Read the model definition and answer for the solid it produces. Units are mm, in the model's axes. Round coordinates to 2 decimals unless told otherwise and drop trailing zeros. Order: outer loops, then holes, each group sorted by start corner. A loop starts at its lowest first (then second) coordinate and runs counter-clockwise, first axis right, second up. Notation, with made-up numbers: (-4.5, 32) - (52.5, 32) arc R16 cw to (52.5, 45) - close; hole circle Ø9 at (-38, 81.25). An arc over 180 degrees is marked (long way). One line per question, with ' | ' between items. Start each with the question number.
1) The part is cut by section B-B, the plane z = -5. Give the vertices of the cut face in (x, y), plus the area to 3 significant figures.
2) The part is cut by section A-A, the plane x = 15.5. Give the vertices of the cut face in (y, z), plus the area to 3 significant figures.
3) Straight lines are drawn through the part: line 1 (X direction, y = 1.2, z = 9); line 2 (X direction, y = 1.65, z = 8); line 3 (X direction, y = 2.55, z = -1.25). For each, find the intervals that lie inside material, in ascending order. Write a range as from..to.
4) The mould has two halves that part along Z. Classify faces 1 (the cylindrical face through (15.56, 2.03, -6.45)), 2 (the flat face through (-17, 2, -12.5)), 3 (the flat face through (-25, 2, 1)): pulls with the +Z half, pulls with the -Z half, needs draft (parallel to the pull), parting line crosses it, or undercut.
5) The part is cut by section C-C, the plane y = 3.35. Give the vertices of the cut face in (x, z).
6) The part is cut by section D-D, the plane z = -10. Give the vertices of the cut face in (x, y), plus the area to 3 significant figures.
from build123d import *

# Parameters (mm, degrees)
SKETCH_1_W          = 50
SKETCH_1_H          = 25
EXTRUDE_1_DEPTH     = 4
SKETCH_2_R          = 1.45
CUT_EXTRUDE_1_DEPTH = 4
SKETCH_3_R          = 12.5
CUT_EXTRUDE_2_DEPTH = 4
SKETCH_5_W          = 50
SKETCH_5_H          = 4
EXTRUDE_2_DEPTH     = 3
FILLET_1_R          = 4
SKETCH_11_R         = 1.5
CUT_EXTRUDE_4_DEPTH = 10


with BuildPart() as part:
    # 草图1 → 凸台-拉伸1 (new body)
    with BuildSketch(Plane(origin=(0, 0, 0), x_dir=(1, 0, 0), z_dir=(0, 1, 0))):
        Rectangle(SKETCH_1_W, SKETCH_1_H)
    extrude(amount=EXTRUDE_1_DEPTH)

    # 草图2 → 切除-拉伸1 (cut)
    with BuildSketch(Plane(origin=(0, 4, 0), x_dir=(1, 0, 0), z_dir=(0, 1, 0))):
        with Locations(Location((-15.5, 5, 0), (0, 0, 270))):
            Circle(SKETCH_2_R)
        with Locations(Location((15.5, 5, 0), (0, 0, 270))):
            Circle(SKETCH_2_R)
    extrude(amount=-CUT_EXTRUDE_1_DEPTH, mode=Mode.SUBTRACT)

    # 草图3 → 切除-拉伸2 (cut)
    with BuildSketch(Plane(origin=(0, 4, 0), x_dir=(1, 0, 0), z_dir=(0, 1, 0))):
        with Locations((0, 12.5)):
            Circle(SKETCH_3_R)
    extrude(amount=-CUT_EXTRUDE_2_DEPTH, mode=Mode.SUBTRACT)

    # 草图5 → 凸台-拉伸2 (add)
    with BuildSketch(Plane.XY.offset(12.5)):
        with Locations((0, 2)):
            Rectangle(SKETCH_5_W, SKETCH_5_H)
    extrude(amount=EXTRUDE_2_DEPTH)

    # 圆角1
    fillet_1_edges = [part.edges().sort_by_distance(p)[0] for p in [
        (-25, 2, 15.5),
        (25, 2, 15.5),
        (-25, 2, -12.5),
        (25, 2, -12.5),
    ]]
    fillet(fillet_1_edges, radius=FILLET_1_R)

    # 草图11 → 切除-拉伸4 (cut)
    with BuildSketch(Plane(origin=(0, 4, 0), x_dir=(1, 0, 0), z_dir=(0, 1, 0))):
        with Locations(Location((-15.5, -9, 0), (0, 0, 270))):
            Circle(SKETCH_11_R)
        with Locations(Location((15.5, -9, 0), (0, 0, 270))):
            Circle(SKETCH_11_R)
    extrude(amount=-CUT_EXTRUDE_4_DEPTH, mode=Mode.SUBTRACT)


solid = part.part
Values:
1) outline: (-25, 0) - (-16.95, 0) - (-16.95, 4) - (-25, 4) - close; (-14.05, 0) - (-10, 0) - (-10, 4) - (-14.05, 4) - close; (10, 0) - (14.05, 0) - (14.05, 4) - (10, 4) - close; (16.95, 0) - (25, 0) - (25, 4) - (16.95, 4) - close | area: 96.8 mm^2
2) outline: (0, -12.5) - (4, -12.5) - (4, -6.45) - (0, -6.45) - close; (0, -3.55) - (4, -3.55) - (4, 7.5) - (0, 7.5) - close; (0, 10.5) - (4, 10.5) - (4, 15.5) - (0, 15.5) - close | area: 88.4 mm^2
3) line 1: x = -25..-17, -14..14, 17..25 | line 2: x = -25..-16.62, -14.38..14.38, 16.62..25 | line 3: x = -25..-5.45, 5.45..25
4) face 1: undercut | face 2: pulls with the -Z half | face 3: needs draft
5) outline: (-25, -8.5) arc R4 ccw to (-21, -12.5) - (-12.5, -12.5) arc R12.5 cw to (12.5, -12.5) - (21, -12.5) arc R4 ccw to (25, -8.5) - (25, 11.5) arc R4 ccw to (21, 15.5) - (-21, 15.5) arc R4 ccw to (-25, 11.5) - close; hole circle Ø3 at (-15.5, 9); hole circle Ø2.9 at (-15.5, -5); hole circle Ø3 at (15.5, 9); hole circle Ø2.9 at (15.5, -5)
6) outline: (-24.71, 0) - (-12.25, 0) - (-12.25, 4) - (-24.71, 4) - close; (12.25, 0) - (24.71, 0) - (24.71, 4) - (12.25, 4) - close | area: 99.7 mm^2
